```python
from build123d import *

# Parameters (mm, degrees)
SKETCH1_R                = 4.5
BOSS_EXTRUDE1_DEPTH      = 2.5
SKETCH2_W                = 10
SKETCH2_H                = 45
BOSS_EXTRUDE2_DEPTH      = 5
CUT_EXTRUDE1_DEPTH       = 147.126229678
CUT_EXTRUDE1_DEPTH_BACK  = 147.126229678
BOSS_EXTRUDE3_DEPTH      = 12.05
FILLET1_R                = 5
FILLET2_R                = 5
BOSS_EXTRUDE4_DEPTH      = 10
BOSS_EXTRUDE4_DEPTH_BACK = 2.000004
SKETCH6_W                = 30.1
SKETCH6_H                = 156
SKETCH6_W_2              = 24.1
SKETCH6_H_2              = 150
BOSS_EXTRUDE5_DEPTH      = 5
SKETCH8_W                = 30.1
SKETCH8_H                = 121
BOSS_EXTRUDE6_DEPTH      = 3
CUT_EXTRUDE2_REACH       = 179.268
SKETCH10_W               = 24.1
SKETCH10_H               = 15
SKETCH11_W               = 0.2
SKETCH11_H               = 2.7
BOSS_EXTRUDE7_DEPTH      = 153


with BuildPart() as part:
    # Sketch1 → Boss-Extrude1 (new, symmetric)
    with BuildSketch(Plane(origin=(0, 0, 0), x_dir=(1, 0, 0), z_dir=(0, 1, 0))):
        with BuildLine():
            Line((-31.821067812, 7.071067812), (-7.071067812, 31.821067812))
            ThreePointArc((-7.071067812, 31.821067812), (0, 34.75), (7.071067812, 31.821067812))
            Line((7.071067812, 31.821067812), (31.821067812, 7.071067812))
            ThreePointArc((31.821067812, 7.071067812), (34.75, 0), (31.821067812, -7.071067812))
            Line((31.821067812, -7.071067812), (7.071067812, -31.821067812))
            ThreePointArc((7.071067812, -31.821067812), (0, -34.75), (-7.071067812, -31.821067812))
            Line((-7.071067812, -31.821067812), (-31.821067812, -7.071067812))
            ThreePointArc((-31.821067812, -7.071067812), (-34.75, 0), (-31.821067812, 7.071067812))
        make_face()
        with Locations(Location((0, 24.75, 0), (0, 0, 270))):
            Circle(SKETCH1_R, mode=Mode.SUBTRACT)
        with Locations(Location((24.75, 0, 0), (0, 0, 270))):
            Circle(SKETCH1_R, mode=Mode.SUBTRACT)
        with Locations(Location((0, -24.75, 0), (0, 0, 270))):
            Circle(SKETCH1_R, mode=Mode.SUBTRACT)
        with Locations(Location((-24.75, 0, 0), (0, 0, 270))):
            Circle(SKETCH1_R, mode=Mode.SUBTRACT)
    extrude(amount=BOSS_EXTRUDE1_DEPTH, both=True)


with BuildPart() as body_2:
    # Mirror3: mirrored copy
    add(part.part.mirror(Plane.XY.offset(49.5)))


with BuildPart() as body_3:
    # Sketch2 → Boss-Extrude2 (new, symmetric)
    with BuildSketch(Plane(origin=(0, 0, 0), x_dir=(0, 0, -1), z_dir=(1, 0, 0))):
        with Locations((-99, 25)):
            Rectangle(SKETCH2_W, SKETCH2_H)
    extrude(amount=BOSS_EXTRUDE2_DEPTH, both=True)


with BuildPart() as body_4:
    # Mirror5: mirrored copy
    add(body_3.part.mirror(Plane.XY.offset(49.5)))


with BuildPart() as cut_extrude1_tool:
    # Sketch3 → Cut-Extrude1 (new, two sides: drawn at the far end of the back side and taken through both)
    with BuildSketch(Plane(origin=(0, 0, 0), x_dir=(0, 0, -1), z_dir=(1, 0, 0)).offset(-CUT_EXTRUDE1_DEPTH_BACK)):
        Polygon((-398.060619113, -61.293305417), (-104, 17.5), (5, 46.706461975), (299.060619113, 125.499767392), (141.474008279, 713.621005618), (-555.647229947, 526.827932809), align=None)
    extrude(amount=CUT_EXTRUDE1_DEPTH + CUT_EXTRUDE1_DEPTH_BACK)


with BuildPart() as body_3_1:
    add(body_3.part)

    # Cut-Extrude1: cut by cut_extrude1_tool
    add(cut_extrude1_tool.part, mode=Mode.SUBTRACT)


with BuildPart() as body_4_1:
    add(body_4.part)

    # Cut-Extrude1: cut by cut_extrude1_tool
    add(cut_extrude1_tool.part, mode=Mode.SUBTRACT)

    # Combine2: union part
    add(part.part)

    # Fillet2
    fillet2_edges = [body_4_1.edges().sort_by_distance(p)[0] for p in [
        (-5, 2.5, 0),
        (0, 2.5, 5),
        (0, 2.5, -5),
        (5, 2.5, 0),
    ]]
    fillet(fillet2_edges, radius=FILLET2_R)


with BuildPart() as body_5:
    # Sketch4 → Boss-Extrude3 (new, symmetric)
    with BuildSketch(Plane(origin=(0, 0, 0), x_dir=(0, 0, -1), z_dir=(1, 0, 0))):
        Polygon((-130.821067812, 10.31331654), (14.067806131, 49.136173305), (13.550168041, 51.068024958), (-131.338705902, 12.245168192), align=None)
    extrude(amount=BOSS_EXTRUDE3_DEPTH, both=True)



with BuildPart() as body_2_1:
    add(body_2.part)

    # Combine1: union body 3
    add(body_3_1.part)

    # Fillet1
    fillet1_edges = [body_2_1.edges().sort_by_distance(p)[0] for p in [
        (0, 2.5, 94),
        (5, 2.5, 99),
        (-5, 2.5, 99),
        (0, 2.5, 104),
    ]]
    fillet(fillet1_edges, radius=FILLET1_R)


with BuildPart() as body_5_1:
    add(body_5.part)

    add(body_2_1.part)  # Boss-Extrude4 merges body 2

    add(body_4_1.part)  # Boss-Extrude4 merges body 4
    # Sketch6 → Boss-Extrude4 (add, two sides: drawn at the far end of the back side and taken through both)
    with BuildSketch(Plane(origin=(0, 44.259573936, 11.859317093), x_dir=(1, 0, 0), z_dir=(0, 0.96592582628907, 0.2588190451025143)).offset(-BOSS_EXTRUDE4_DEPTH_BACK)):
        with Locations((0, -48.694165284)):
            Rectangle(SKETCH6_W, SKETCH6_H)
        with Locations((0, -48.694165284)):
            Rectangle(SKETCH6_W_2, SKETCH6_H_2, mode=Mode.SUBTRACT)
    extrude(amount=BOSS_EXTRUDE4_DEPTH + BOSS_EXTRUDE4_DEPTH_BACK)

    # Sketch7 → Boss-Extrude5 (add)
    with BuildSketch(Plane(origin=(0, 53.918832199, 14.447507544), x_dir=(1, 0, 0), z_dir=(0, 0.96592582628907, 0.25881904510251436))):
        Polygon((12.05, 26.305834716), (12.05, -91.694165284), (15.05, -91.694165284), (15.05, 29.305834716), (-15.05, 29.305834716), (-15.05, -91.694165284), (-12.05, -91.694165284), (-12.05, 26.305834716), align=None)
    extrude(amount=BOSS_EXTRUDE5_DEPTH)

    # Sketch8 → Boss-Extrude6 (add)
    with BuildSketch(Plane(origin=(0, 58.74846133, 15.74160277), x_dir=(1, 0, 0), z_dir=(0, 0.96592582628907, 0.25881904510251436))):
        with Locations((0, -31.194165284)):
            Rectangle(SKETCH8_W, SKETCH8_H)
    extrude(amount=BOSS_EXTRUDE6_DEPTH)

    # Sketch10 → Cut-Extrude2 (cut, up to next)
    with BuildSketch(Plane(origin=(0, 6.808451022, -25.409485135), x_dir=(1, 0, 0), z_dir=(0, -0.2588190451025143, 0.96592582628907)), mode=Mode.PRIVATE) as cut_extrude2_sk1:
        with Locations((0, 53.320882651)):
            Rectangle(SKETCH10_W, SKETCH10_H)
    cut_extrude2_tool1 = extrude(cut_extrude2_sk1.sketch, amount=-CUT_EXTRUDE2_REACH, mode=Mode.PRIVATE) & body_5_1.part
    add(cut_extrude2_tool1.solids().sort_by_distance((0, 58.312469, -11.609025))[0], mode=Mode.SUBTRACT)

    # Sketch11 → Boss-Extrude7 (add)
    with BuildSketch(Plane(origin=(0, 7.584908157, -28.307262614), x_dir=(-1, 0, 0), z_dir=(0, 0.2588190451025143, -0.96592582628907))):
        with Locations((-11.95, 47.170882651)):
            Rectangle(SKETCH11_W, SKETCH11_H)
        with Locations((11.95, 47.170882651)):
            Rectangle(SKETCH11_W, SKETCH11_H)
    extrude(amount=-BOSS_EXTRUDE7_DEPTH)


solid = body_5_1.part
```
The listing builds one solid part. Answer for the finished solid, in the listing's coordinates (mm). A direction names the side the tool comes from. Round coordinates to 2 decimals unless told otherwise and drop trailing zeros. Write each loop counter-clockwise with the first axis right and the second up, starting at its lowest first coordinate (ties: lowest second). Pieces come first, ordered by that corner, then holes. Notation, with made-up numbers: (67.25, -17.75) -> (114.25, -17.75) arc R22 ccw to (114.25, 7.25) -> close; hole circle Ø6 at (26, 37.25). An arc over 180 degrees is marked (long way). Answer as a JSON object with one key per item and string values. Group by question number.
Q1. Section B-B (x = 24.75) is taken. Write down the section's boundary in (y, z), plus the area to 3 significant figures.
Q2. Section D-D (y = 59) is taken. Write down the section's boundary in (x, z), plus the area to 3 significant figures.
Q3. Determine the mould class of faces 5 (the face through (0.11, 0.04, 64.25)), 6 (the face through (-7.18, 3.37, 0.14)), 7 (the face through (0, 27, -5)), 8 (the face through (11.85, 34, 57)) for opening direction Z: pulls with the +Z half, pulls with the -Z half, needs draft (parallel to the pull), parting line crosses it, or undercut.
Q4. Which of the six approach directions +Z, -Z, +X, -X, +Y, -Y give full straight-line access (tool end or side, diameter ignored) to faces 1 (the face through (0, 14, 94)), 2 (the face through (19.62, 0.04, 79.73)), 3 (the face through (0.198, -0.035, 128.246)), 4 (the face through (-12.05, 40, 61))?
Q5. Each of these flat-tipped pins is pushed along its axis until it touches: pin 1 Ø5.5 at (x, z) = (0, 74.25) entering from -Y; pin 2 Ø3 at (y, z) = (12.5, 100.5) entering from +X; pin 3 Ø14.5 at (x, z) = (0, 123.75) entering from -Y; pin 4 Ø3 at (x, z) = (-4, 2) entering from +Y. Where does it stop, or does it pass through?
Q6. Section A-A (z = 24.75) is taken. Count the separate pieces of the cut face and the enclosed holes in it, plus the area to 3 significant figures.
Q7. Straight lines are drawn through the part: line 1 along X through (y, z) = (46, 27.5); line 2 along X through (y, z) = (-0.5, 99); line 3 along Z through (x, y) = (-24, 0). For each, find the intervals that lie inside material, in ascending order.
Check values:
{
 "1": {"outline": "(-2.5, -14.14) -> (2.5, -14.14) -> (2.5, -4.5) -> (-2.5, -4.5) -> close; (-2.5, 4.5) -> (2.5, 4.5) -> (2.5, 14.14) -> (-2.5, 14.14) -> close; (-2.5, 84.86) -> (2.5, 84.86) -> (2.5, 94.5) -> (-2.5, 94.5) -> close; (-2.5, 103.5) -> (2.5, 103.5) -> (2.5, 113.14) -> (-2.5, 113.14) -> close", "area": "193 mm^2"},
 "2": {"outline": "(-15.05, -14.53) -> (-12.05, -14.53) -> (-12.05, 14.8) -> (12.05, 14.8) -> (12.05, -14.53) -> (15.05, -14.53) -> (15.05, 26.39) -> (-15.05, 26.39) -> close", "area": "525 mm^2"},
 "3": {"face 5": "undercut", "face 6": "needs draft", "face 7": "pulls with the -Z half", "face 8": "undercut"},
 "4": {"face 1": "+X, -X", "face 2": "+X, -Y", "face 3": "-Y", "face 4": "none"},
 "5": {"pin 1": "y = 24.73", "pin 2": "x = 5", "pin 3": "y = -2.5", "pin 4": "y = 65.94"},
 "6": {"separate pieces": "3", "enclosed holes": "1", "area": "347 mm^2"},
 "7": {"line 1": "-15.05 to -12.05, 12.05 to 15.05", "line 2": "-34.75 to -29.25, -20.25 to 20.25, 29.25 to 34.75", "line 3": "-14.89 to -4.44, 4.44 to 14.89, 84.11 to 94.56, 103.44 to 113.89"}
}
